Verification items for the finished model (mm, model axes). Round coordinates to 2 decimals unless told otherwise and drop trailing zeros. Write each loop counter-clockwise with the first axis right and the second up, starting at its lowest first coordinate (ties: lowest second). Pieces come first, ordered by that corner, then holes. Notation, with made-up numbers: (71, -40) - (111, -40) arc R27 ccw to (111, -5) - close; hole circle Ø1 at (4.25, 82). An arc over 180 degrees is marked (long way). Answer as a JSON object with one key per item and string values.
```python
from build123d import *

# Parameters (mm, degrees)
F0_W     = 146.05
F0_H     = 76.2
F2_DEPTH = 76.2
F3_R     = 20.887507
F4_DEPTH = 76.2
F1_W     = 25.4
F1_H     = 25.4
F5_DEPTH = 76.2


with BuildPart() as f2:
    # F0 (on Front) → F2 (new body)
    with BuildSketch(Plane.XZ):
        with Locations((-20.51247, 13.275895)):
            Rectangle(F0_W, F0_H)
    extrude(amount=F2_DEPTH)

    # F3 (on face) → F4 (cut)
    with BuildSketch(Plane.XZ):
        with Locations((28.185513, 16.4221)):
            Circle(F3_R)
    extrude(amount=F4_DEPTH, mode=Mode.SUBTRACT)

    # F1 (on face) → F5 (join)
    with BuildSketch(Plane.XZ):
        with Locations((-52.30484, 12.7)):
            Rectangle(F1_W, F1_H)
    extrude(amount=F5_DEPTH)


solid = f2.part
```
1. Go/stop test with a flat-tipped pin: pin 1 (10 mm diameter, centred on x = -73, z = 11, fed in from +Y). Record where the tip stops, or that it passes through.
Completed:
{"pin 1": "stops at y = 0"}
2. Cross-section at B-B (x = 19). Record the boundary of the cut face in (y, z).
Completed:
{"outline": "(-76.2, -24.82) - (0, -24.82) - (0, -2.34) - (-76.2, -2.34) - close; (-76.2, 35.18) - (0, 35.18) - (0, 51.38) - (-76.2, 51.38) - close"}
3. Cross-section at A-A (z = 30). Record the boundary of the cut face in (x, y), plus the area to 3 significant figures.
Completed:
{"outline": "(-93.54, -76.2) - (12.31, -76.2) - (12.31, 0) - (-93.54, 0) - close; (44.06, -76.2) - (52.51, -76.2) - (52.51, 0) - (44.06, 0) - close", "area": "8,710 mm^2"}
4. Mould release check, pull along X, two halves, no side actions. Record for faces 1 (the face through (-93.537, -38, 13)), 2 (the face through (23.66, -37.57, -3.97)), 3 (the face through (-22, -38, -24.824)): released by +X, released by -X, zero draft, split by the parting line, or undercut.
Completed:
{"face 1": "released by -X", "face 2": "undercut", "face 3": "zero draft"}
5. Cross-section at C-C (y = -27.5). Record the boundary of the cut face in (x, z), plus the area to 3 significant figures.
Completed:
{"outline": "(-93.54, -24.82) - (52.51, -24.82) - (52.51, 51.38) - (-93.54, 51.38) - close; hole circle Ø41.78 at (28.19, 16.42)", "area": "9,760 mm^2"}
6. Material ranges on probe 1 along Z at (x, y) = (28, -10.5); probe 2 along X at (y, z) = (-41.5, 27.5); probe 3 along Z at (x, y) = (32.5, -72), recorded low to high. Write a range as from..to.
Completed:
{"probe 1": "z = -24.82..-4.46, 37.31..51.38", "probe 2": "x = -93.54..10.48, 45.89..52.51", "probe 3": "z = -24.82..-4.01, 36.86..51.38"}
